Source: three-view drawing plus pictorial views. Frame: mm from the lowest corner of the part. Give positions to 0.01 mm unless a question says otherwise; leave off trailing zeros. Loops run counter-clockwise (first coordinate to the right, second up) from the corner with the lowest first, then second, coordinate; pieces in that order, holes last.
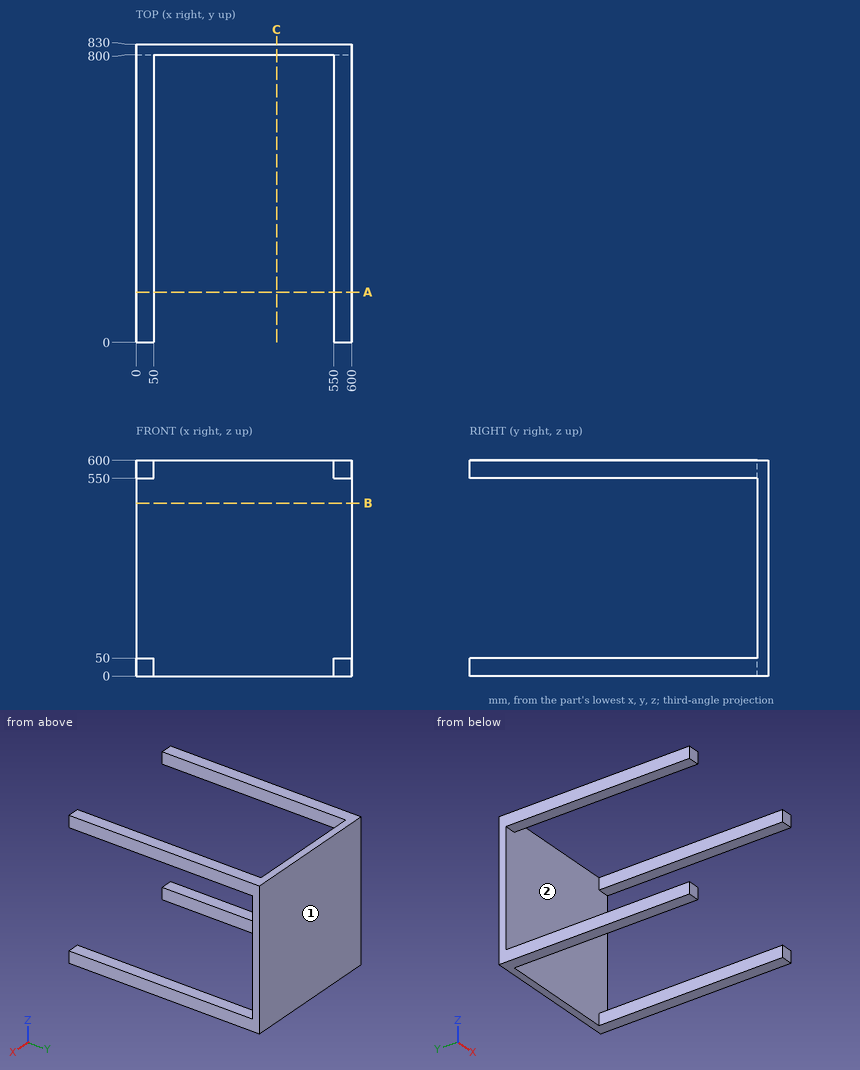
Q1. Mould query, pull axis X, two halves, no side actions, for the marked faces 1 and 2. Classes: +X half, -X half, draft (parallel to the pull), parting line (faces both ways), or undercut.
Q2. Pin query (flat end, axial travel): pin 1 Ø5 at (x, z) = (209, 386.5) entering from -Y. Return the tip coordinate at first contact, or that it passes through.
Q3. Section query B-B, the plane z = 481. Return loops of the section in (x, y), and give its area (3 significant figures).
Q4. Section query A-A, the plane y = 140. Return loops of the section in (x, z), and give its area (3 significant figures).
Q5. Section query C-C, the plane x = 391.5. Return loops of the section in (y, z), and give its area (3 significant figures).
Q6. Material intervals for probe 1 along Z at (x, y) = (35.5, 169); probe 2 along Y at (x, z) = (115, 305), sorted ascending.
Resolved:
1. face 1: draft
1. face 2: undercut
2. pin 1: stops at y = 800
3. outline: (0, 800) - (600, 800) - (600, 830) - (0, 830) - close
3. area: 18,000 mm2
4. outline: (0, 0) - (50, 0) - (50, 50) - (0, 50) - close; (0, 550) - (50, 550) - (50, 600) - (0, 600) - close; (550, 0) - (600, 0) - (600, 50) - (550, 50) - close; (550, 550) - (600, 550) - (600, 600) - (550, 600) - close
4. area: 10,000 mm2
5. outline: (800, 0) - (830, 0) - (830, 600) - (800, 600) - close
5. area: 18,000 mm2
6. probe 1: z = 0 to 50, 550 to 600
6. probe 2: y = 800 to 830
